from build123d import *

# Parameters (mm, degrees)
BOSS_EXTRUDE1_DEPTH = 6.35
SKETCH2_R           = 2.25
CUT_EXTRUDE1_DEPTH  = 5
SKETCH3_R           = 2.25
CUT_EXTRUDE2_DEPTH  = 5


with BuildPart() as part:
    # Sketch1 → Boss-Extrude1 (new body)
    with BuildSketch(Plane.XY):
        Polygon((0, 0), (0, 43), (15, 43), (43, 15), (43, 0), align=None)
        Polygon((38, 5), (5, 5), (5, 38), (12.928932188, 38), (38, 12.928932188), align=None, mode=Mode.SUBTRACT)
    extrude(amount=BOSS_EXTRUDE1_DEPTH)

    # Sketch2 → Cut-Extrude1 (cut)
    with BuildSketch(Plane.XZ):
        with Locations((16, 3.175)):
            Circle(SKETCH2_R)
        with Locations((24, 3.175)):
            Circle(SKETCH2_R)
        with Locations((32, 3.175)):
            Circle(SKETCH2_R)
    extrude(amount=-CUT_EXTRUDE1_DEPTH, mode=Mode.SUBTRACT)

    # Sketch3 → Cut-Extrude2 (cut)
    with BuildSketch(Plane.ZY):
        with Locations((3.175, 16)):
            Circle(SKETCH3_R)
        with Locations((3.175, 24)):
            Circle(SKETCH3_R)
        with Locations((3.175, 32)):
            Circle(SKETCH3_R)
    extrude(amount=-CUT_EXTRUDE2_DEPTH, mode=Mode.SUBTRACT)


solid = part.part
For this review, take the finished solid that the model builds, in its own axes (mm). A direction names the side the tool comes from. Give positions to 0.01 mm unless a question says otherwise; leave off trailing zeros. Loops run counter-clockwise (first coordinate to the right, second up) from the corner with the lowest first, then second, coordinate; pieces in that order, holes last.
Item 1: For line 1 along Z through (x, y) = (16, 1.15) (3 decimals); line 2 along Y through (x, z) = (9, 3.5); line 3 along Y through (x, z) = (3.5, 3.25), list the stretches that pass through material, from the lowest coordinate up.
Item 2: Take a section at A-A, the plane y = 8. State the section outline as (x, z) points.
Item 3: Draft analysis for pull direction Z (two halves, no side actions). For faces 1 (the flat face through (43, 8, 3)), 2 (the cylindrical face through (2.46, 33.9, 4.38)), 3 (the flat face through (27, 27, 0)), state which applies: +Z half, -Z half, draft (parallel to the pull), parting line (faces both ways), or undercut.
Item 4: Tool access review of faces 4 (the flat face through (29, 29, 3)), 5 (the cylindrical face through (26.146, 2.465, 3.851)), 6 (the flat face through (9, 38, 3)), 7 (the cylindrical face through (2.5, 21.8, 2.7)), 8 (the flat face through (27, 27, 6.35)): name each direction out of +Z, -Z, +X, -X, +Y, -Y from which nothing blocks a thin tool from reaching the whole face with its end or side.
Item 5: Insertion check: pin 1 (2 mm diameter, centred on x = 18, z = 4.5, fed in from +Y); pin 2 (4 mm diameter, centred on x = 35.5, y = 11, fed in from +Z); pin 3 (3.5 mm diameter, centred on x = 24, z = 3.175, fed in from +Y); pin 4 (2.5 mm diameter, centred on y = 24, z = 3.175, fed in from -X). Each pin has a flat end and moves straight along its axis. Give the tip position at first contact, or say it passes through.
Item 6: Take a section at D-D, the plane z = 1.5. Give the number of separate pieces and of enclosed holes in the cut face, and give its area (3 significant figures).
Item 7: Take a section at B-B, the plane x = 24. State the section outline as (y, z) points (3 decimals).
Calculated:
1. line 1: z = 0 to 0.925, 5.425 to 6.35
1. line 2: y = 0 to 5, 38 to 43
1. line 3: y = 0 to 13.75, 18.25 to 21.75, 26.25 to 29.75, 34.25 to 43
2. outline: (0, 0) - (5, 0) - (5, 6.35) - (0, 6.35) - close; (38, 0) - (43, 0) - (43, 6.35) - (38, 6.35) - close
3. face 1: draft
3. face 2: undercut
3. face 3: -Z half
4. face 4: +Z, -Z, +X, +Y
4. face 5: -Y
4. face 6: +Z, -Z
4. face 7: -X
4. face 8: +Z, +X, -X, +Y, -Y
5. pin 1: stops at y = 41
5. pin 2: passes through
5. pin 3: stops at y = 35.75
5. pin 4: stops at x = 25.68
6. separate pieces: 6
6. enclosed holes: 0
6. area: 592 mm2
7. outline: (0, 0) - (5, 0) - (5, 0.925) - (0, 0.925) - close; (0, 5.425) - (5, 5.425) - (5, 6.35) - (0, 6.35) - close; (26.929, 0) - (34, 0) - (34, 6.35) - (26.929, 6.35) - close
